The listing builds one solid part. Answer for the finished solid, in the listing's coordinates (mm). Give positions to 0.01 mm unless a question says otherwise; leave off trailing zeros. Order: outer loops, then holes, each group sorted by start corner. A loop starts at its lowest first (then second) coordinate and runs counter-clockwise, first axis right, second up.
```python
from build123d import *

# Parameters (mm, degrees)
BOSS_EXTRUDE1_DEPTH = 3.175
SKETCH3_R           = 2.38125
CUT_EXTRUDE2_DEPTH  = 3.175


with BuildPart() as part:
    # Sketch1 → Boss-Extrude1 (new body)
    with BuildSketch(Plane.XY):
        Polygon((-3.175, 365.778475051), (-34.925, 365.778475051), (-34.925, 342.421386502), (-38.1, 342.421386502), (-38.1, 323.371386502), (-34.925, 323.371386502), (-34.925, 298.240631325), (-38.1, 298.240631325), (-38.1, 279.190631325), (-34.925, 279.190631325), (-34.925, 267.318840011), (-3.175, 267.318840011), (-3.175, 279.190631325), (0, 279.190631325), (0, 298.240631325), (-3.175, 298.240631325), (-3.175, 323.371386502), (0, 323.371386502), (0, 342.421386502), (-3.175, 342.421386502), align=None)
    extrude(amount=BOSS_EXTRUDE1_DEPTH)

    # Sketch3 → Cut-Extrude2 (cut)
    with BuildSketch(Plane.XY.offset(3.175)):
        with Locations((-19.05, 316.548657531)):
            Circle(SKETCH3_R)
        with BuildLine():
            ThreePointArc((-6.700444288, 328.898213243), (-19.05, 334.013566708), (-31.399555712, 328.898213243))
            ThreePointArc((-31.399555712, 328.898213243), (-31.399555712, 325.530617198), (-28.031959666, 325.530617198))
            ThreePointArc((-28.031959666, 325.530617198), (-19.05, 329.251066708), (-10.068040334, 325.530617198))
            ThreePointArc((-10.068040334, 325.530617198), (-6.700444288, 325.530617198), (-6.700444288, 328.898213243))
        make_face()
        with BuildLine():
            ThreePointArc((-31.397852166, 304.200805365), (-19.05, 299.086157531), (-6.702147834, 304.200805365))
            ThreePointArc((-6.702147834, 304.200805365), (-6.702147834, 307.56840141), (-10.069743879, 307.56840141))
            ThreePointArc((-10.069743879, 307.56840141), (-19.05, 303.848657531), (-28.030256121, 307.56840141))
            ThreePointArc((-28.030256121, 307.56840141), (-31.397852166, 307.56840141), (-31.397852166, 304.200805365))
        make_face()
    extrude(amount=-CUT_EXTRUDE2_DEPTH, mode=Mode.SUBTRACT)


solid = part.part
```
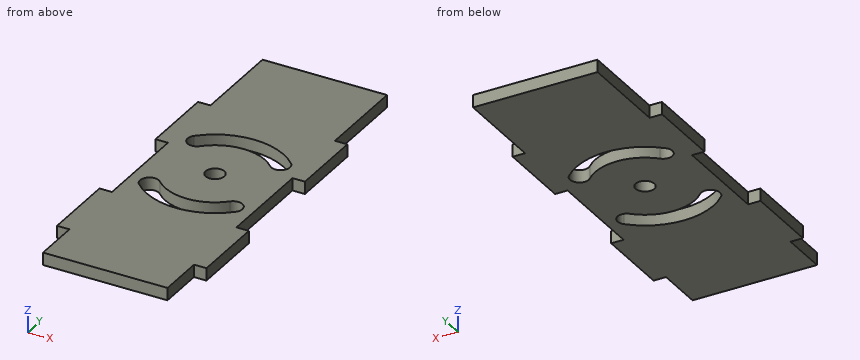
1) Find section B-B (z = 0.75). Count the separate pieces of the cut face and the enclosed holes in it, then the cut area to 3 significant figures.
Geometry says:
separate pieces: 1
enclosed holes: 3
area: 3,090 mm2
2) Straight lines are drawn through the part: probe 1 along Y at (x, z) = (-19.05, 1.85); probe 2 along Y at (x, z) = (-17, 2.7); probe 3 along Y at (x, z) = (-11.5, 1.5). For each, find the intervals that lie inside material, in ascending order.
Geometry says:
probe 1: y = 267.32 to 299.09, 303.85 to 314.17, 318.93 to 329.25, 334.01 to 365.78
probe 2: y = 267.32 to 299.21, 304.02 to 315.34, 317.76 to 329.08, 333.89 to 365.78
probe 3: y = 267.32 to 300.8, 306.34 to 326.76, 332.3 to 365.78
3) Find section C-C (x = -30.5). Write down the section's boundary in (y, z) (3 decimals).
Geometry says:
outline: (267.319, 0) - (303.364, 0) - (303.364, 3.175) - (267.319, 3.175) - close; (308.132, 0) - (324.966, 0) - (324.966, 3.175) - (308.132, 3.175) - close; (329.737, 0) - (365.778, 0) - (365.778, 3.175) - (329.737, 3.175) - close
4) Find section A-A (x = -19.05). Write down the section's boundary in (y, z) (3 decimals).
Geometry says:
outline: (267.319, 0) - (299.086, 0) - (299.086, 3.175) - (267.319, 3.175) - close; (303.849, 0) - (314.167, 0) - (314.167, 3.175) - (303.849, 3.175) - close; (318.93, 0) - (329.251, 0) - (329.251, 3.175) - (318.93, 3.175) - close; (334.014, 0) - (365.778, 0) - (365.778, 3.175) - (334.014, 3.175) - close
5) Find section D-D (y = 356.5). Write down the section's boundary in (x, z) (3 decimals), then the cut area to 3 significant figures.
Geometry says:
outline: (-34.925, 0) - (-3.175, 0) - (-3.175, 3.175) - (-34.925, 3.175) - close
area: 101 mm2
6) Given P1, Ø1.6, axis at y = 273.5, z = 1.5, coming from the +X side (3 decimals); P2, Ø1.6, axis at x = -1, z = 1, coming from the +Y side; P3, Ø1, axis at x = -1, z = 1, coming from the -Y side, each flat-ended and moving along its own axis, determine where each tip first touches the part or whether it passes through.
Geometry says:
P1: stops at x = -3.175
P2: stops at y = 342.42
P3: stops at y = 279.19
